Input: part model. Units: mm. Frame: model coordinates. Face numbers are marked on the shaded views. A direction names the side the tool comes from. Give positions to 0.01 mm unless a question says otherwise; leave off trailing zeros. Write each loop counter-clockwise with the first axis right and the second up, starting at its lowest first coordinate (ties: lowest second). Pieces come first, ordered by that corner, then holes. Notation, with made-up numbers: (7, -35.75) - (50, -35.75) arc R32 ccw to (50, -0.75) - close; hole circle Ø3 at (44.25, 78). An arc over 180 degrees is marked (long way). Use a Markdown table: item, result. Add a question column.
1. Pin query (flat end, axial travel): pin 1 (2 mm diameter, centred on y = -1, z = -11.5, fed in from -X); pin 2 (1 mm diameter, centred on x = -2, y = -1.5, fed in from -Z); pin 3 (2 mm diameter, centred on x = 0, y = 0, fed in from +Z). Return the tip coordinate at first contact, or that it passes through.
2. Section query C-C, the plane z = -4.25. Return loops of the section in (x, y).
3. Section query B-B, the plane y = 0. Return loops of the section in (x, z).
4. Mould query, pull axis Y, two halves, no side actions, for the marked faces 1, 2 and 3. Classes: released by +Y, released by -Y, zero draft, split by the parting line, or undercut.
5. Section query D-D, the plane x = 2.4. Return loops of the section in (y, z), plus the area to 3 significant figures.
6. Material intervals for probe 1 along Z at (x, y) = (-1, 0); probe 2 along Z at (x, y) = (-1.65, 1.75); probe 3 along X at (y, z) = (-0.5, -1.5), sorted ascending.
7. Section query A-A, the plane z = -10. Return loops of the section in (x, y), plus the area to 3 significant figures.
8. Set-up query: the marked faces 4 and 5. Return all of +Z, -Z, +X, -X, +Y, -Y with unobstructed straight access to the full face (end or side cutting, diameter ignored); none if empty.
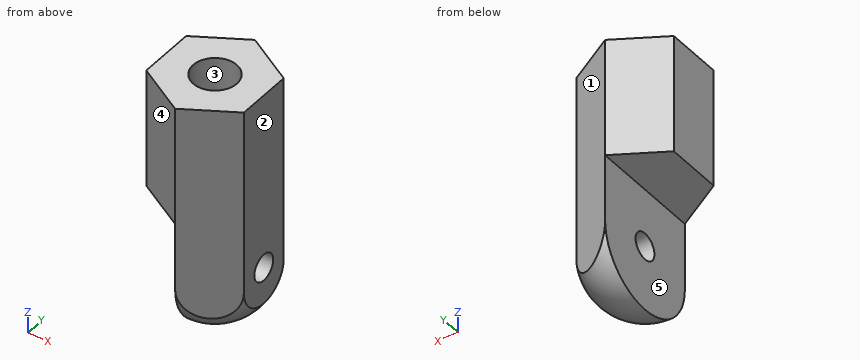
```python
from build123d import *

# Parameters (mm, degrees)
AUFSATZ_LINEAR_AUSTRAGEN1_DEPTH      = 15
SKIZZE1_3_OUTSIDE_W                  = 10.938
SKIZZE1_3_OUTSIDE_H                  = 11.788
SKIZZE1_3_OUTSIDE_R                  = 1.23
SCHNITT_LINEAR_AUSTRAGEN3_DEPTH      = 6
SKIZZE3_R                            = 0.75
SCHNITT_LINEAR_AUSTRAGEN1_DEPTH      = 6.5
SKIZZE4_W                            = 2.75
SKIZZE4_H                            = 6.975426481
SCHNITT_LINEAR_AUSTRAGEN2_DEPTH      = 4.175426481
SCHNITT_LINEAR_AUSTRAGEN2_DEPTH_BACK = 4.175426481


with BuildPart() as part:
    # Skizze1 → Aufsatz-Linear austragen1 (new body)
    with BuildSketch(Plane.XY):
        Polygon((-2.75, 1.58771324), (-2.75, -1.58771324), (0, -3.175426481), (2.75, -1.58771324), (2.75, 1.58771324), (0, 3.175426481), align=None)
    extrude(amount=-AUFSATZ_LINEAR_AUSTRAGEN1_DEPTH)

    # Skizze1_3 outside → Schnitt-Linear austragen3 (cut)
    with BuildSketch(Plane.XY):
        Rectangle(SKIZZE1_3_OUTSIDE_W, SKIZZE1_3_OUTSIDE_H)
        Polygon((-2.75, 1.58771324), (-2.75, -1.58771324), (0, -3.175426481), (2.75, -1.58771324), (2.75, 1.58771324), (0, 3.175426481), align=None, mode=Mode.SUBTRACT)
        Circle(SKIZZE1_3_OUTSIDE_R)
    extrude(amount=-SCHNITT_LINEAR_AUSTRAGEN3_DEPTH, mode=Mode.SUBTRACT)

    # Skizze2 → Schnitt-Rotation1 (revolve, cut)
    with BuildSketch(Plane(origin=(0, 0, 0), x_dir=(0, 0, -1), z_dir=(1, 0, 0))):
        with BuildLine():
            Line((10.5, 3.175426481), (10.5, 5))
            Line((10.5, 5), (15, 5))
            Line((15, 5), (15, 0))
            Line((15, 0), (13.675426481, 0))
            ThreePointArc((13.675426481, 0), (12.745365598, 2.245365598), (10.5, 3.175426481))
        make_face()
    revolve(axis=Axis((0, 0, 0), (0, 0, -1)), mode=Mode.SUBTRACT)

    # Skizze3 → Schnitt-Linear austragen1 (cut, through all)
    with BuildSketch(Plane(origin=(2.75, 0, 0), x_dir=(0, 0, -1), z_dir=(1, 0, 0))):
        with Locations((10, 0)):
            Circle(SKIZZE3_R)
    extrude(amount=-SCHNITT_LINEAR_AUSTRAGEN1_DEPTH, mode=Mode.SUBTRACT)

    # Skizze4 → Schnitt-Linear austragen2 (cut, two sides)
    with BuildSketch(Plane(origin=(0, 0, 0), x_dir=(1, 0, 0), z_dir=(0, 1, 0))) as schnitt_linear_austragen2_sk:
        with Locations((-1.375, 10.187713241)):
            Rectangle(SKIZZE4_W, SKIZZE4_H)
    extrude(amount=SCHNITT_LINEAR_AUSTRAGEN2_DEPTH, mode=Mode.SUBTRACT)
    extrude(schnitt_linear_austragen2_sk.sketch, amount=-SCHNITT_LINEAR_AUSTRAGEN2_DEPTH_BACK, mode=Mode.SUBTRACT)


solid = part.part
```
Result sheet:
| question | item | result |
|---|---|---|
| 1 | pin 1 | stops at x = 0 |
| 1 | pin 2 | stops at z = -6.7 |
| 1 | pin 3 | stops at z = -6 |
| 2 | outline | (-2.75, -1.59) - (0, -3.18) - (2.75, -1.59) - (2.75, 1.59) - (0, 3.18) - (-2.75, 1.59) - close; hole circle Ø2.46 at (0, 0) |
| 3 | outline | (-2.75, -6.7) - (0, -6.7) - (0, -9.25) - (2.75, -9.25) - (2.75, 0) - (1.23, 0) - (1.23, -6) - (-1.23, -6) - (-1.23, 0) - (-2.75, 0) - close; (0, -13.68) arc R3.18 ccw to (2.75, -12.09) - (2.75, -10.75) - (0, -10.75) - close |
| 4 | face 1 | released by +Y |
| 4 | face 2 | zero draft |
| 4 | face 3 | undercut |
| 5 | outline | (-1.79, -11.56) arc R2.08 ccw to (1.79, -11.56) - (1.79, 0) - (-1.79, 0) - close; hole circle Ø1.5 at (0, -10) |
| 5 | area | 42.2 mm² |
| 6 | probe 1 | z = -6.7 to -6 |
| 6 | probe 2 | z = -6.7 to 0 |
| 6 | probe 3 | x = -2.75 to -1.12, 1.12 to 2.75 |
| 7 | outline | (0, -3.18) - (2.75, -1.59) - (2.75, -0.75) - (0, -0.75) - close; (0, 0.75) - (2.75, 0.75) - (2.75, 1.59) - (0, 3.18) - close |
| 7 | area | 8.97 mm² |
| 8 | face 4 | +Z, -Z, -X, -Y |
| 8 | face 5 | -Z, -X, +Y, -Y |
